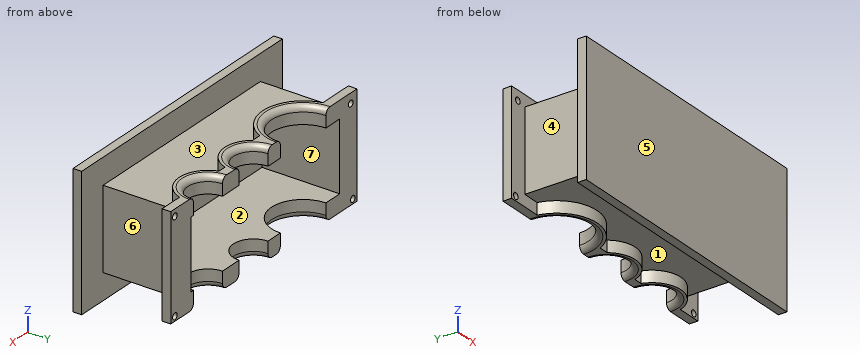
Autodesk Inventor part; units mm, degrees
ref_plane "Work Plane1" through (0, 0, -60) normal (0, 0, -1) x (-1, 0, 0)
ref_plane "YZ Plane" through (0, 0, 0) normal (1, 0, 0) x (0, 1, 0)
ref_plane "XZ Plane" through (0, 0, 0) normal (0, 1, 0) x (-1, 0, 0)
sketch "Sketch1" plane through (0, 0, 0) normal (0, 0, 1) x (1, 0, 0)
  arc A0 (-55, 0) -> (55, 0) centre (0, 0) ccw
  arc A1 (-70, 0) -> (63.2456, -30) centre (0, 0) ccw
  arc A2 (85, 0) -> (155, 0) centre (120, 0) ccw
  arc A3 (80, -30) -> (167.697, -15) centre (120, 0) ccw
  arc A4 (195, 0) -> (265, 0) centre (230, 0) ccw
  arc A5 (182.303, -15) -> (277.697, -15) centre (230, 0) ccw
  line L0 (-130, 0) -> (-130, -15)
  line L1 (320, -15) -> (320, 0)
  line L2 (-130, -15) -> (-68.374, -15)
  line L3 (-130, 0) -> (-55, 0)
  line L4 (63.2456, -30) -> (80, -30)
  line L5 (167.697, -15) -> (182.303, -15)
  line L6 (277.697, -15) -> (320, -15)
  line L7 (265, 0) -> (320, 0)
  line L8 (55, 0) -> (85, 0)
  line L9 (155, 0) -> (195, 0)
  line L10 (-98.374, -15) -> (-98.374, -145)
  line L11 (-98.374, -145) -> (281.626, -145)
  line L12 (281.626, -145) -> (281.626, -15)
  dimension "d0" = 110
  dimension "d1" = 140
  dimension "d2" = 70
  dimension "d3" = 100
  dimension "d4" = 70
  dimension "d5" = 100
  dimension "d10" = 15
  dimension "d12" = 130
  dimension "d70" = 120
  dimension "d71" = 110
  dimension "d72" = 380
  dimension "d75" = 130
  dimension "d76" = 30
  dimension "d77" = 15
  dimension "d92" = 450
extrude "Extrusion1" add sketch "Sketch1" along normal blind 30 contours A0 L8 A2 L9 A4 L7 L1 L6 A5 L5 A3 L4 A1 L3 | A1 L2 L0 L3
extrude "Extrusion2" add sketch "Sketch1" along normal blind 10 contours A1 L4 A3 L5 A5 L6 L12 L11 L10 L2
sketch "Sketch2" plane through (0, 0, 0) normal (0, 0, -1) x (-1, 0, 0)
  line L0 (-281.626, -145) -> (-281.626, -15)
  line L1 (98.374, -145) -> (-281.626, -145)
  line L2 (98.374, -15) -> (98.374, -145)
  line L3 (-271.626, -15) -> (-271.626, -135)
  line L4 (-271.626, -135) -> (88.374, -135)
  line L5 (88.374, -135) -> (88.374, -15)
  line L6 (-281.626, -15) -> (-320, -15)
  line L7 (130, -15) -> (98.374, -15)
  line L8 (-281.626, -15) -> (-271.626, -15)
  line L9 (88.374, -15) -> (98.374, -15)
  point P0 (0, 0)
  dimension "d19" = 10
extrude "Extrusion3" add sketch "Sketch2" along normal blind 130
ref_plane "Work Plane1" through (0, 0, -60) normal (0, 0, -1) x (-1, 0, 0)
mirror "Mirror1" about plane through (0, 0, -60) normal (0, 0, -1) of "Extrusion1", "Extrusion2"
sketch "Sketch3" plane through (0, 0, -60) normal (0, 0, -1) x (-1, 0, 0)
  line L0 (88.374, -135) -> (88.374, -15)
  line L1 (130, 0) -> (130, -15)
  line L2 (88.374, -15) -> (130, -15)
  line L3 (130, -15) -> (130, 0)
  line L4 (130, 0) -> (88.374, 0)
  line L5 (88.374, 0) -> (88.374, -15)
  line L6 (-271.626, -15) -> (-271.626, -135)
  line L7 (-320, 0) -> (-265, 0)
  line L8 (-271.626, -15) -> (-320, -15)
  line L9 (-320, -15) -> (-320, 0)
  line L10 (-320, 0) -> (-271.626, 0)
  line L11 (-271.626, 0) -> (-271.626, -15)
  point P0 (0, 0)
  point P1 (-271.626, 0)
extrude "Extrusion4" add sketch "Sketch3" along normal through all both and the other way through all
sketch "Sketch4" plane through (0, 0, -60) normal (0, 0, -1) x (-1, 0, 0)
  line L0 (-281.626, -15) -> (-281.626, -145)
  line L1 (-333.586, -145) -> (151.414, -145)
  line L2 (151.414, -145) -> (151.414, -160)
  line L3 (151.414, -160) -> (-333.586, -160)
  line L4 (-333.586, -145) -> (-333.586, -160)
  point P0 (0, 0)
  dimension "d29" = 51.96
  dimension "d30" = 485
  dimension "d31" = 15
extrude "Extrusion5" add sketch "Sketch4" along normal mid plane 230
fillet "Fillet1" radius 10 6 edges at (0, -55, 30) (120, -35, 30) (230, -35, 30) (230, -35, -150) (120, -35, -150) (0, -55, -150)
sketch "Sketch9" plane through (-130, -15, 30) normal (0, -1, 0) x (1, 0, 0)
  point P0 (15, -17)
hole "Hole5" at (-115, -15, 13) direction (0, 1, 0) diameter 11 depth 15
sketch "Sketch10" plane through (-130, -15, 30) normal (0, -1, 0) x (1, 0, 0)
  point P0 (10, -172)
hole "Hole6" at (-120, -15, -142) direction (0, 1, 0) diameter 11 depth 15
sketch "Sketch11" plane through (277.697, -15, 30) normal (0, -1, 0) x (1, 0, 0)
  point P0 (32.303, -172)
hole "Hole7" at (310, -15, -142) direction (0, 1, 0) diameter 11 depth 15
sketch "Sketch12" plane through (277.697, -15, 30) normal (0, -1, 0) x (1, 0, 0)
  point P0 (32.303, -12)
hole "Hole8" at (310, -15, 18) direction (0, 1, 0) diameter 11 depth 15
Build history of the part. All positions in model axes, mm. Face numbers are marked on the shaded views. A direction names the side the tool comes from. Round coordinates to 2 decimals unless told otherwise and drop trailing zeros. Order: outer loops, then holes, each group sorted by start corner. A loop starts at its lowest first (then second) coordinate and runs counter-clockwise, first axis right, second up. Notation, with made-up numbers: M 24.25,-9 L 81.25,-9 A20 cw 81.25,26 Z; hole C 0,45.5 d2. An arc over 180 degrees is marked long. Use CSV: the item, a comma, the result in double quotes. Start each with the question number.
(1) Flat gauge pins, fed straight in: P1, Ø16.5, axis at y = -7.5, z = -37.5, coming from the +X side; P2, Ø3, axis at y = -60, z = -132.5, coming from the -X side; P3, Ø6, axis at x = -71, y = -109, coming from the -Z side. Where does each tip first touch, or does it go through?
(2) Cut at C-C on z = -26.5. List the corners of the cut face in (x, y).
(3) Cut at A-A on x = 310. List the corners of the cut face in (y, z), then the cut area to 3 significant figures.
(4) Cut at B-B on y = -124.5. List the corners of the cut face in (x, z).
(5) Drill centre lines: probe 1 along Z at (x, y) = (310, -12); probe 2 along X at (y, z) = (-4, -142); probe 3 along Y at (x, z) = (295.5, -132.5). Where is each one in solid material? Low to high.
(6) Mould opens along Z. For the marked faces 1, 2, 3 and 4 say: +Z half, -Z half, draft (parallel to the pull), parting line (faces both ways), or undercut.
(7) Cut at D-D on x = 0. List the corners of the cut face in (y, z).
(8) Tool access for the marked faces 5, 6 and 7: list every direction of +Z, -Z, +X, -X, +Y, -Y with a clear straight run to the whole face (end or side of a thin tool).
Findings:
1,P1,"stops at x = 320"
1,P2,"stops at x = -38.44"
1,P3,"stops at z = -130"
2,outline,"M -151.41,-160 L 333.59,-160 L 333.59,-145 L 281.63,-145 L 281.63,-15 L 320,-15 L 320,0 L 271.63,0 L 271.63,-135 L -88.37,-135 L -88.37,0 L -130,0 L -130,-15 L -98.37,-15 L -98.37,-145 L -151.41,-145 Z"
3,outline,"M -160,-175 L -145,-175 L -145,55 L -160,55 Z; M -15,-150 L 0,-150 L 0,-147.5 L -15,-147.5 Z; M -15,-136.5 L 0,-136.5 L 0,12.5 L -15,12.5 Z; M -15,23.5 L 0,23.5 L 0,30 L -15,30 Z"
3,area,"5,820 mm^2"
4,outline,"M -98.37,-130 L 281.63,-130 L 281.63,10 L -98.37,10 Z; hole M -88.37,-120 L 271.63,-120 L 271.63,0 L -88.37,0 Z"
5,probe 1,"z = -150 to -147.5, -136.5 to 12.5, 23.5 to 30"
5,probe 2,"x = -130 to -125.5, -114.5 to -55.06, 55.06 to 85.03, 154.97 to 195.03, 264.97 to 304.5, 315.5 to 320"
5,probe 3,"y = -160 to -145, -15 to 0"
6,face 1,"-Z half"
6,face 2,"undercut"
6,face 3,"+Z half"
6,face 4,"draft"
7,outline,"M -160,-175 L -145,-175 L -145,-130 L -70,-130 L -70,-150 L -65,-150 A10 ccw -55,-140 L -55,-120 L -135,-120 L -135,0 L -55,0 L -55,20 A10 ccw -65,30 L -70,30 L -70,10 L -145,10 L -145,55 L -160,55 Z"
8,face 5,"+Z, -Z, +X, -X, -Y"
8,face 6,"+Z, -Z, +X"
8,face 7,"+Y"
